from build123d import *

# Parameters (mm, degrees)
SKETCH2_R          = 2.794
EXTRUDE1_DEPTH     = 7.62
CUT_EXTRUDE1_DEPTH = 9.583546586
LPATTERN1_COUNT    = 2
LPATTERN1_PITCH    = 8.001
EXTRUDE3_DEPTH     = 7.62
FILLET1_R          = 2.54


with BuildPart() as part:
    # Sketch2 → Extrude1 (new body)
    with BuildSketch(Plane.XY):
        with Locations(Location((0, 0, 0), (0, 0, 180))):
            Circle(SKETCH2_R)
    extrude(amount=EXTRUDE1_DEPTH)

    # Sketch3 → Cut-Extrude1 (cut, through all)
    with BuildSketch(Plane.XY.offset(7.62)):
        with BuildLine():
            Line((-0.762, 2.032), (-0.762, 1.016))
            ThreePointArc((-0.762, 1.016), (-0.836394878, 0.836394878), (-1.016, 0.762))
            Line((-1.016, 0.762), (-2.032, 0.762))
            ThreePointArc((-2.032, 0.762), (-2.211605122, 0.687605122), (-2.286, 0.508))
            Line((-2.286, 0.508), (-2.286, -0.508))
            ThreePointArc((-2.286, -0.508), (-2.211605122, -0.687605122), (-2.032, -0.762))
            Line((-2.032, -0.762), (-1.016, -0.762))
            ThreePointArc((-1.016, -0.762), (-0.836394878, -0.836394878), (-0.762, -1.016))
            Line((-0.762, -1.016), (-0.762, -2.032))
            ThreePointArc((-0.762, -2.032), (-0.687605122, -2.211605122), (-0.508, -2.286))
            Line((-0.508, -2.286), (0.508, -2.286))
            ThreePointArc((0.508, -2.286), (0.687605122, -2.211605122), (0.762, -2.032))
            Line((0.762, -2.032), (0.762, -1.016))
            ThreePointArc((0.762, -1.016), (0.836394878, -0.836394878), (1.016, -0.762))
            Line((1.016, -0.762), (2.032, -0.762))
            ThreePointArc((2.032, -0.762), (2.211605122, -0.687605122), (2.286, -0.508))
            Line((2.286, -0.508), (2.286, 0.508))
            ThreePointArc((2.286, 0.508), (2.211605122, 0.687605122), (2.032, 0.762))
            Line((2.032, 0.762), (1.016, 0.762))
            ThreePointArc((1.016, 0.762), (0.836394878, 0.836394878), (0.762, 1.016))
            Line((0.762, 1.016), (0.762, 2.032))
            ThreePointArc((0.762, 2.032), (0.687605122, 2.211605122), (0.508, 2.286))
            Line((0.508, 2.286), (-0.508, 2.286))
            ThreePointArc((-0.508, 2.286), (-0.687605122, 2.211605122), (-0.762, 2.032))
        make_face()
    extrude(amount=-CUT_EXTRUDE1_DEPTH, mode=Mode.SUBTRACT)


with BuildPart() as lpattern1_1:
    # LPattern1: pattern copy
    add(part.part.moved(Location(Vector(1, 0, 0) * (1 * LPATTERN1_PITCH))))


with BuildPart() as part_1:
    add(part.part)

    add(lpattern1_1.part)  # Extrude3 merges LPattern1_1
    # Sketch5 → Extrude3 (add, through all)
    with BuildSketch(Plane.XY.offset(7.62)):
        with BuildLine():
            Line((2.286, 1.797323066), (2.286, -1.797323066))
            ThreePointArc((2.286, -1.797323066), (4.0005, -1.338121812), (5.715, -1.797323066))
            Line((5.715, -1.797323066), (5.715, 1.797323066))
            ThreePointArc((5.715, 1.797323066), (4.0005, 1.338121812), (2.286, 1.797323066))
        make_face()
    extrude(amount=-EXTRUDE3_DEPTH)

    # Fillet1
    # the kernel refuses this fillet: 2.54 mm, written as the material it adds along each edge
    with BuildSketch(Plane(origin=(2.286, 1.606437051, 7.62), x_dir=(-0.6706382745586644, 0.7417845406160589, 0), z_dir=(0, 0, -1))) as fillet1_piece_1:
        with BuildLine():
            CenterArc((0.993305965, 2.520961484), FILLET1_R, 250.408076785, 12.572378174)
            Line((0.141596295, 0.128015467), (0, 0))
            ThreePointArc((0, 0), (0.341448925, 0.020942368), (0.682897851, 0))
        make_face()
    extrude(amount=7.62)
    with BuildSketch(Plane(origin=(2.286, -1.606437051, 7.62), x_dir=(-0.6706382745586632, -0.7417845406160598, 0), z_dir=(0, 0, -1))) as fillet1_piece_2:
        with BuildLine():
            CenterArc((0.993305965, -2.520961484), FILLET1_R, 97.019545041, 12.572378174)
            Line((0.141596295, -0.128015467), (0, 0))
            ThreePointArc((0, 0), (0.341448925, -0.020942368), (0.682897851, 0))
        make_face()
    extrude(amount=7.62)
    with BuildSketch(Plane(origin=(5.715, -1.606437051, 7.62), x_dir=(0, -1, 0), z_dir=(0, 0, -1))) as fillet1_piece_3:
        with BuildLine():
            CenterArc((2.427472269, 1.203861258), FILLET1_R, 208.291730517, 12.572378174)
            ThreePointArc((0.506563069, -0.457977436), (0.267326288, -0.213453994), (0, 0))
            Line((0, 0), (0.190886015, 0))
        make_face()
    extrude(amount=7.62)
    with BuildSketch(Plane(origin=(5.715, 1.606437051, 7.62), x_dir=(0, 1, 0), z_dir=(0, 0, -1))) as fillet1_piece_4:
        with BuildLine():
            CenterArc((2.427472269, -1.203861258), FILLET1_R, 139.135891309, 12.572378174)
            ThreePointArc((0.506563069, 0.457977436), (0.267326288, 0.213453994), (0, 0))
            Line((0, 0), (0.190886015, 0))
        make_face()
    extrude(amount=7.62)


solid = part_1.part
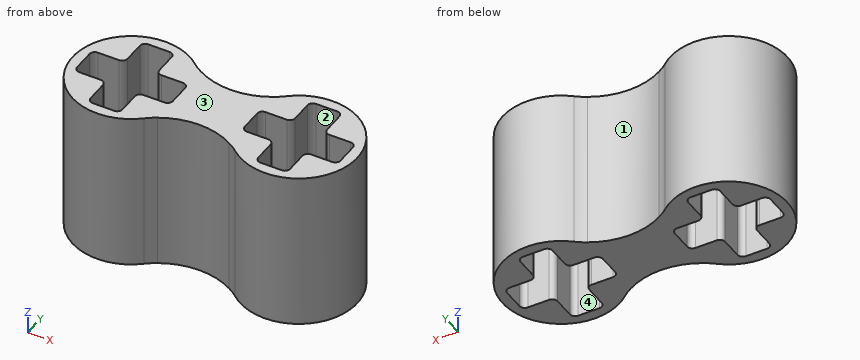
Model file for the job. Use its own axes, mm. Face numbers are marked on the shaded views. A direction names the side the tool comes from. Round coordinates to 2 decimals unless told otherwise and drop trailing zeros. Order: outer loops, then holes, each group sorted by start corner. A loop starts at its lowest first (then second) coordinate and runs counter-clockwise, first axis right, second up.
(1) Band-saw the part on B-B (x = 0). List the corners of the cut face in (y, z).
(2) 3-axis set-ups, long thin cutter, end or side, ignore diameter. For the marked faces 1 and 2: which of +Z, -Z, +X, -X, +Y, -Y reach the whole face in a straight line?
(3) Band-saw the part on D-D (z = 2.5). Give the number of separate pieces and of enclosed holes in the cut face, then the cut area to 3 significant figures.
(4) Drill centre lines: line 1 (X direction, y = 0.1, z = 1.5) (3 decimals); line 2 (X direction, y = -2.1, z = 2); line 3 (X direction, y = -2.2, z = 7.25). Where is each one in solid material? Low to high.
(5) Band-saw the part on A-A (y = 0). List the corners of the cut face in (x, z) (3 decimals), then the cut area to 3 significant figures.
(6) Band-saw the part on C-C (y = 1.65). List the corners of the cut face in (x, z), then the cut area to 3 significant figures.
(7) Pin check, flat tips, straight feed: pin 1 (0.5 mm diameter, centred on x = 10, z = 5, fed in from +Y); pin 2 (1.1 mm diameter, centred on y = 1.5, z = 4.5, fed in from -X); pin 3 (0.5 mm diameter, centred on x = 9.5, z = 3, fed in from -Y). Stop position of each tip, or through.
(8) Pull direction X, two halves, no side cores. Call the marked faces 3 and 4: released by +X, released by -X, zero draft, split by the parting line, or undercut.
Verdict:
1. outline: (-2.79, 0) - (-2.29, 0) - (-2.29, 7.62) - (-2.79, 7.62) - close; (2.29, 0) - (2.79, 0) - (2.79, 7.62) - (2.29, 7.62) - close
2. face 1: +Z, -Z, +Y
2. face 2: +Z, -Z
3. separate pieces: 1
3. enclosed holes: 2
3. area: 34.0 mm2
4. line 1: x = -2.792 to -2.286, 2.286 to 5.715, 10.287 to 10.793
4. line 2: x = -1.84 to -0.75, 0.75 to 1.84, 6.16 to 7.25, 8.75 to 9.84
4. line 3: x = -1.72 to -0.7, 0.7 to 1.72, 6.28 to 7.3, 8.7 to 9.72
5. outline: (-2.794, 0) - (-2.286, 0) - (-2.286, 7.62) - (-2.794, 7.62) - close; (2.286, 0) - (5.715, 0) - (5.715, 7.62) - (2.286, 7.62) - close; (10.287, 0) - (10.795, 0) - (10.795, 7.62) - (10.287, 7.62) - close
5. area: 33.9 mm2
6. outline: (-2.25, 0) - (-0.76, 0) - (-0.76, 7.62) - (-2.25, 7.62) - close; (0.76, 0) - (2.57, 0) - (2.57, 7.62) - (0.76, 7.62) - close; (5.43, 0) - (7.24, 0) - (7.24, 7.62) - (5.43, 7.62) - close; (8.76, 0) - (10.26, 0) - (10.26, 7.62) - (8.76, 7.62) - close
6. area: 50.3 mm2
7. pin 1: stops at y = 2.18
7. pin 2: stops at x = -2.63
7. pin 3: stops at y = -2.5
8. face 3: zero draft
8. face 4: undercut
